Study the drawing (mm; zero at the part's minimum x, y, z) and answer. Coordinates: 2 decimals unless noted, no trailing zeros. Order: outer loops, then holes, each group sorted by start corner. A loop starts at its lowest first (then second) coordinate and runs counter-clockwise, first axis right, second up.
1. Flat-ended cylindrical pins translate along their axes: pin 1 Ø3 at (x, z) = (4.2, 31) entering from +Y; pin 2 Ø1 at (y, z) = (1.5, 13.5) entering from -X. Find the tip coordinate at first contact, or state that the pin passes through.
2. Find the intervals of material crossed by probe 1 along Z at (x, y) = (31, 1.5); probe 2 along Z at (x, y) = (3.5, 0.2) (1 decimal); probe 3 along Z at (x, y) = (6.5, 0.95) (1 decimal), in increasing order.
3. The part is cut by section A-A, the plane z = 31. Give the vertices of the cut face in (x, y).
4. The part is cut by section B-B, the plane x = 31. Give the vertices of the cut face in (y, z).
5. The part is cut by section D-D, the plane y = 1.1. Give the vertices of the cut face in (x, z).
6. The part is cut by section C-C, the plane z = 20. Give the vertices of the cut face in (x, y).
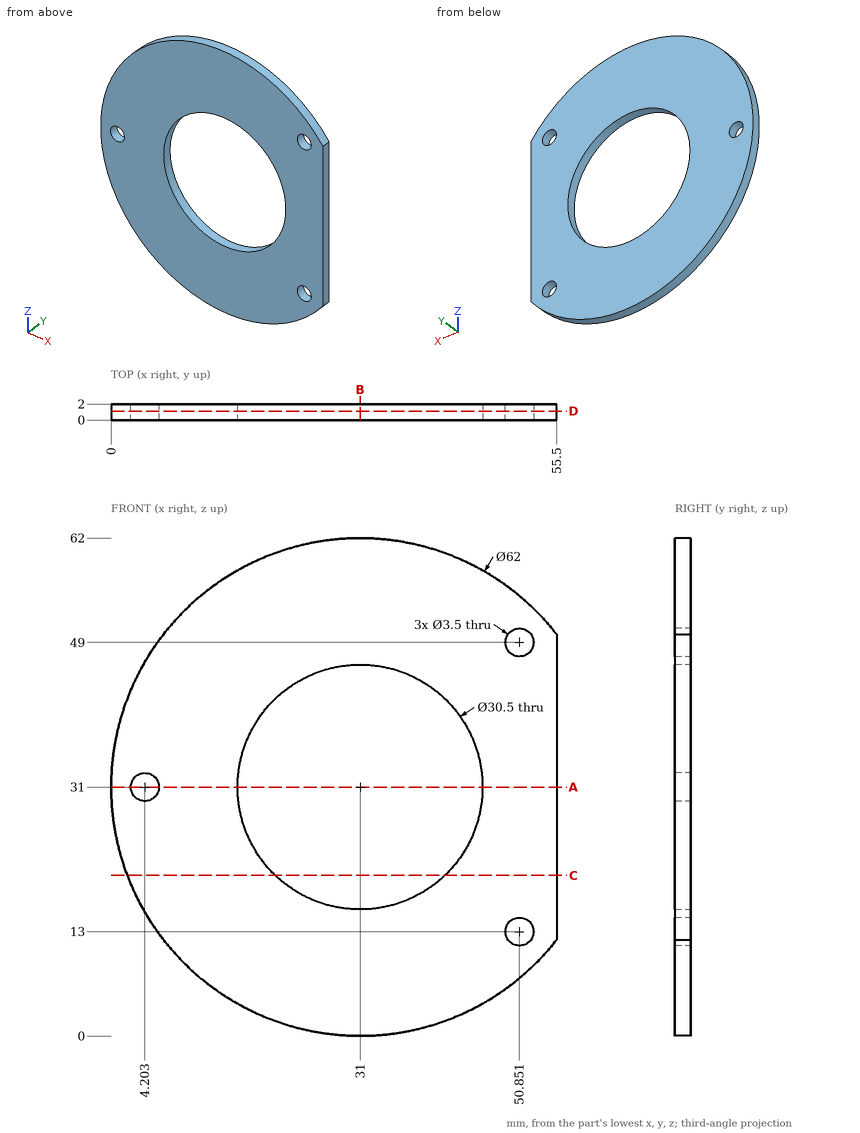
Geometry says:
1. pin 1: passes through
1. pin 2: stops at x = 5.08
2. probe 1: z = 0 to 15.75, 46.25 to 62
2. probe 2: z = 16.7 to 29.4, 32.6 to 45.3
2. probe 3: z = 12 to 50
3. outline: (0, 0) - (2.45, 0) - (2.45, 2) - (0, 2) - close; (5.95, 0) - (15.75, 0) - (15.75, 2) - (5.95, 2) - close; (46.25, 0) - (55.5, 0) - (55.5, 2) - (46.25, 2) - close
4. outline: (0, 0) - (2, 0) - (2, 15.75) - (0, 15.75) - close; (0, 46.25) - (2, 46.25) - (2, 62) - (0, 62) - close
5. outline: (55.5, 12.01) - (55.5, 49.99) arc R31 ccw (long way) to start; hole circle Ø3.5 at (4.2, 31); hole circle Ø30.5 at (31, 31); hole circle Ø3.5 at (50.85, 13); hole circle Ø3.5 at (50.85, 49)
6. outline: (2.02, 0) - (20.44, 0) - (20.44, 2) - (2.02, 2) - close; (41.56, 0) - (55.5, 0) - (55.5, 2) - (41.56, 2) - close
